Verification items for the finished model (mm, model axes). Coordinates: 2 decimals unless noted, no trailing zeros. Order: outer loops, then holes, each group sorted by start corner. A loop starts at its lowest first (then second) coordinate and runs counter-clockwise, first axis right, second up. Notation, with made-up numbers: M 33.5,1.25 L 76.5,1.25 A29 cw 76.5,27.25 Z; hole C -13.75,-13 d6. An arc over 180 degrees is marked long. Answer as a JSON object with one key per item and string values. Group by question number.
(1) Mould release check, pull along Z, two halves, no side actions. Record for faces 1 (the face through (8.779, 10.846, -13.686)), 2 (the face through (0, 11, 15)), 3 (the face through (17, 8, 4)): released by +Z, released by -Z, zero draft, split by the parting line, or undercut.
(2) Cross-section at D-D (z = 0). Enter the section's corners in (x, y).
(3) Material ranges on line 1 (Z direction, x = 9, y = 16.25); line 2 (X direction, y = 14, z = 12); line 3 (Z direction, x = 9, y = 11.25), recorded low to high.
(4) Cross-section at A-A (y = 11). Enter the section's corners in (x, z), plus the area to 3 significant figures.
(5) Cross-section at B-B (z = 12). Enter the section's corners in (x, y), plus the area to 3 significant figures.
(6) Cross-section at C-C (x = 9). Enter the section's corners in (y, z), plus the area to 3 significant figures.
from build123d import *

# Parameters (mm, degrees)
SKETCH1_W           = 34
SKETCH1_H           = 30
SKETCH1_R           = 1.7
BOSS_EXTRUDE1_DEPTH = 22
SKETCH4_R           = 4
CUT_EXTRUDE2_DEPTH  = 42


with BuildPart() as part:
    # Sketch1 → Boss-Extrude1 (new body)
    with BuildSketch(Plane(origin=(0, 0, 0), x_dir=(1, 0, 0), z_dir=(0, 1, 0))):
        Rectangle(SKETCH1_W, SKETCH1_H)
        with Locations((-9, 12)):
            Circle(SKETCH1_R, mode=Mode.SUBTRACT)
        with Locations((9, 12)):
            Circle(SKETCH1_R, mode=Mode.SUBTRACT)
        with Locations((9, -12)):
            Circle(SKETCH1_R, mode=Mode.SUBTRACT)
        with Locations((-9, -12)):
            Circle(SKETCH1_R, mode=Mode.SUBTRACT)
    extrude(amount=BOSS_EXTRUDE1_DEPTH)

    # Sketch4 → Cut-Extrude2 (cut)
    with BuildSketch(Plane(origin=(17, 0, 0), x_dir=(0, 0, -1), z_dir=(1, 0, 0))):
        with Locations((0, 11)):
            Circle(SKETCH4_R)
    extrude(amount=-CUT_EXTRUDE2_DEPTH, mode=Mode.SUBTRACT)


solid = part.part
Taken from the geometry:
{
 "1": {"face 1": "undercut", "face 2": "released by +Z", "face 3": "zero draft"},
 "2": {"outline": "M -17,0 L 17,0 L 17,7 L -17,7 Z; M -17,15 L 17,15 L 17,22 L -17,22 Z"},
 "3": {"line 1": "z = -15 to -13.7, -10.3 to 10.3, 13.7 to 15", "line 2": "x = -17 to -10.7, -7.3 to 7.3, 10.7 to 17", "line 3": "z = -15 to -13.7, -10.3 to -3.99, 3.99 to 10.3, 13.7 to 15"},
 "4": {"outline": "M -17,-15 L 17,-15 L 17,-4 L -17,-4 Z; M -17,4 L 17,4 L 17,15 L -17,15 Z; hole C -9,-12 d3.4; hole C -9,12 d3.4; hole C 9,-12 d3.4; hole C 9,12 d3.4", "area": "712 mm²"},
 "5": {"outline": "M -17,0 L -10.7,0 L -10.7,22 L -17,22 Z; M -7.3,0 L 7.3,0 L 7.3,22 L -7.3,22 Z; M 10.7,0 L 17,0 L 17,22 L 10.7,22 Z", "area": "598 mm²"},
 "6": {"outline": "M 0,-15 L 22,-15 L 22,-13.7 L 0,-13.7 Z; M 0,-10.3 L 22,-10.3 L 22,10.3 L 0,10.3 Z; M 0,13.7 L 22,13.7 L 22,15 L 0,15 Z; hole C 11,0 d8", "area": "460 mm²"}
}
